Input: part model. Units: mm. Frame: model coordinates. Face numbers are marked on the shaded views. A direction names the side the tool comes from. Give positions to 0.01 mm unless a question says otherwise; leave off trailing zeros. Loops run counter-clockwise (first coordinate to the right, second up) from the corner with the lowest first, then second, coordinate; pieces in that order, holes last. Notation, with made-up numbers: (12, -9) -> (39, -9) arc R12 cw to (39, -2) -> close; hole circle Ø3 at (-21.5, 65.25). An arc over 180 degrees is marked (long way). Answer as a JSON object with one key per item and string values. Group by question number.
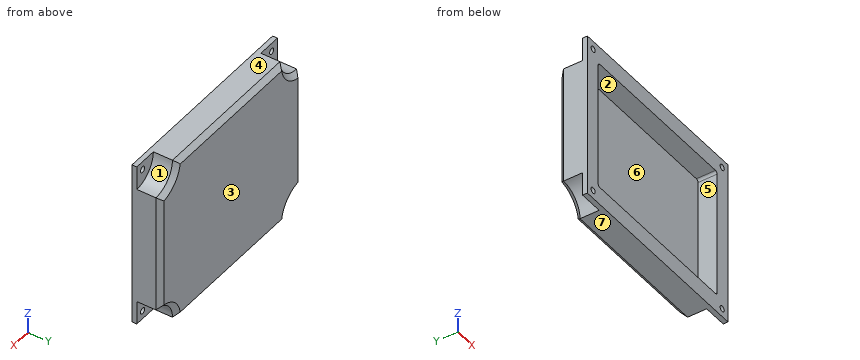
```python
from build123d import *

# Parameters (mm, degrees)
SKETCH2_W                 = 85
SKETCH2_H                 = 70
BOSS_EXTRUDE1_DEPTH       = 12
SKETCH4_R                 = 10
CUT_EXTRUDE3_DEPTH        = 10
FILLET2_SIZE              = 2
M3X0_5_TAPPED_HOLE1_D     = 2.5
M3X0_5_TAPPED_HOLE1_DEPTH = 10
M3X0_5_TAPPED_HOLE1_TIP   = 0.751075774
CUT_EXTRUDE4_DEPTH        = 8


with BuildPart() as part:
    # Sketch2 → Boss-Extrude1 (new body)
    with BuildSketch(Plane(origin=(0, 0, 0), x_dir=(1, 0, 0), z_dir=(0, 1, 0))):
        Rectangle(SKETCH2_W, SKETCH2_H)
    extrude(amount=BOSS_EXTRUDE1_DEPTH)

    # Sketch4 → Cut-Extrude3 (cut)
    with BuildSketch(Plane(origin=(0, 12, 0), x_dir=(1, 0, 0), z_dir=(0, 1, 0))):
        with Locations((42.5, -35)):
            Circle(SKETCH4_R)
        with Locations((-42.5, -35)):
            Circle(SKETCH4_R)
        with Locations((-42.5, 35)):
            Circle(SKETCH4_R)
        with Locations((42.5, 35)):
            Circle(SKETCH4_R)
    extrude(amount=-CUT_EXTRUDE3_DEPTH, mode=Mode.SUBTRACT)

    # Fillet2
    fillet2_edges = [part.edges().sort_by_distance(p)[0] for p in [
        (42.5, 12, 0),
        (0, 12, -35),
        (-42.5, 12, 0),
        (0, 12, 35),
        (35.428932188, 12, -27.928932188),
        (-35.428932188, 12, -27.928932188),
        (-35.428932188, 12, 27.928932188),
        (35.428932188, 12, 27.928932188),
    ]]
    chamfer(fillet2_edges, length=FILLET2_SIZE)

    # M3x0.5 Tapped Hole1
    with Locations(Plane(origin=(0, 2, 0), x_dir=(1, 0, 0), z_dir=(0, 1, 0))):
        with Locations((-39, 31.5), (-39, -31.5), (39, -31.5), (39, 31.5)):
            Hole(M3X0_5_TAPPED_HOLE1_D / 2, depth=M3X0_5_TAPPED_HOLE1_DEPTH)
            with Locations((0, 0, -(M3X0_5_TAPPED_HOLE1_DEPTH + M3X0_5_TAPPED_HOLE1_TIP / 2))):  # 118° drill point
                Cone(0, M3X0_5_TAPPED_HOLE1_D / 2, M3X0_5_TAPPED_HOLE1_TIP, mode=Mode.SUBTRACT)

    # Sketch8 → Cut-Extrude4 (cut)
    with BuildSketch(Plane.XZ):
        with BuildLine():
            Line((35.95, -26.45), (35.95, 26.45))
            ThreePointArc((35.95, 26.45), (35.657106781, 27.157106781), (34.95, 27.45))
            Line((34.95, 27.45), (-34.95, 27.45))
            ThreePointArc((-34.95, 27.45), (-35.657106781, 27.157106781), (-35.95, 26.45))
            Line((-35.95, 26.45), (-35.95, -26.45))
            ThreePointArc((-35.95, -26.45), (-35.657106781, -27.157106781), (-34.95, -27.45))
            Line((-34.95, -27.45), (34.95, -27.45))
            ThreePointArc((34.95, -27.45), (35.657106781, -27.157106781), (35.95, -26.45))
        make_face()
    extrude(amount=-CUT_EXTRUDE4_DEPTH, mode=Mode.SUBTRACT)


solid = part.part
```
Q1. Set-up query: the marked faces 1, 2 and 3. Return all of +Z, -Z, +X, -X, +Y, -Y with unobstructed straight access to the full face (end or side cutting, diameter ignored); none if empty.
Q2. Pin query (flat end, axial travel): pin 1 Ø8 at (x, z) = (-36.5, -31) entering from +Y; pin 2 Ø3 at (x, z) = (25.5, 24) entering from -Y; pin 3 Ø1.5 at (x, z) = (-39, 31.5) entering from +Y; pin 4 Ø3 at (x, z) = (39, 31.5) entering from +Y. Return the tip coordinate at first contact, or that it passes through.
Q3. Section C-C on x = 10. Return the cut outline in (y, z), then the cut area to 3 significant figures.
Q4. Section B-B on z = 3. Return the cut outline in (x, y).
Q5. Pull-direction query (Z, two-part tool) for the marked faces 4, 5, 6 and 7; classes: +Z half, -Z half, draft (parallel to the pull), parting line (faces both ways), or undercut.
Q6. Ray query, probe 1 along X at (y, z) = (1.3, -31.5); probe 2 along Z at (x, y) = (-39, 1.45); probe 3 along Z at (x, y) = (-31, 7.5). Return the intervals inside material, ascending.
Q7. Section D-D on z = -31.5. State how many separate pieces and enclosed holes the cut face has, then the cut area to 3 significant figures.
Q8. Section A-A on y = 7. Return the cut outline in (x, z), then the cut area to 3 significant figures.
Numbers:
{
 "1": {"face 1": "+Z, +X, +Y", "face 2": "-Y", "face 3": "+Z, -Z, +X, -X, +Y"},
 "2": {"pin 1": "stops at y = 11.21", "pin 2": "stops at y = 8", "pin 3": "passes through", "pin 4": "stops at y = 2"},
 "3": {"outline": "(0, -35) -> (10, -35) -> (12, -33) -> (12, 33) -> (10, 35) -> (0, 35) -> (0, 27.45) -> (8, 27.45) -> (8, -27.45) -> (0, -27.45) -> close", "area": "397 mm²"},
 "4": {"outline": "(-42.5, 0) -> (-35.95, 0) -> (-35.95, 8) -> (35.95, 8) -> (35.95, 0) -> (42.5, 0) -> (42.5, 10) -> (40.5, 12) -> (-40.5, 12) -> (-42.5, 10) -> close"},
 "5": {"face 4": "+Z half", "face 5": "undercut", "face 6": "undercut", "face 7": "-Z half"},
 "6": {"probe 1": "x = -42.5 to -40.25, -37.75 to 37.75, 40.25 to 42.5", "probe 2": "z = -35 to -32.75, -30.25 to 30.25, 32.75 to 35", "probe 3": "z = -35 to -27.45, 27.45 to 35"},
 "7": {"separate pieces": "3", "enclosed holes": "0", "area": "818 mm²"},
 "8": {"outline": "(-42.5, -25) arc R10 cw to (-32.5, -35) -> (32.5, -35) arc R10 cw to (42.5, -25) -> (42.5, 25) arc R10 cw to (32.5, 35) -> (-32.5, 35) arc R10 cw to (-42.5, 25) -> close; hole (-35.95, -26.45) arc R1 ccw to (-34.95, -27.45) -> (34.95, -27.45) arc R1 ccw to (35.95, -26.45) -> (35.95, 26.45) arc R1 ccw to (34.95, 27.45) -> (-34.95, 27.45) arc R1 ccw to (-35.95, 26.45) -> close", "area": "1,690 mm²"}
}
